Design review of the part shown in the three views and the two pictorial views. Dimensions are in mm from the part's minimum x, y and z. Coordinates: 2 decimals unless noted, no trailing zeros. Loops run counter-clockwise (first coordinate to the right, second up) from the corner with the lowest first, then second, coordinate; pieces in that order, holes last. Notation, with made-up numbers: (-8, -15) -> (-4, -15) arc R19 cw to (-4, 18) -> close; hole circle Ø3 at (30, -26). An arc over 180 degrees is marked (long way). One line per item, written item: value. Start each with the question number.
1. Add section A-A on x = 2.5. Write out the cut boundary in (y, z) (1 decimal), plus the area to 3 significant figures.
2. Insertion check: pin 1 (2 mm diameter, centred on x = 3, z = 16.5, fed in from +Y); pin 2 (8 mm diameter, centred on x = 17.5, z = 10, fed in from +Y); pin 3 (1.5 mm diameter, centred on x = 4.5, z = 15.5, fed in from -Y). Each pin has a flat end and moves straight along its axis. Give the tip position at first contact, or say it passes through.
3. For probe 1 along Z at (x, y) = (19.5, 18); probe 2 along Z at (x, y) = (8.25, 25); probe 3 along Y at (x, z) = (17, 25) (1 decimal), list the stretches that pass through material, from the lowest coordinate up.
4. Draft analysis for pull direction Z (two halves, no side actions). For the marked faces 1, 2, 3 and 4, state which applies: pulls with the +Z half, pulls with the -Z half, needs draft (parallel to the pull), parting line crosses it, or undercut.
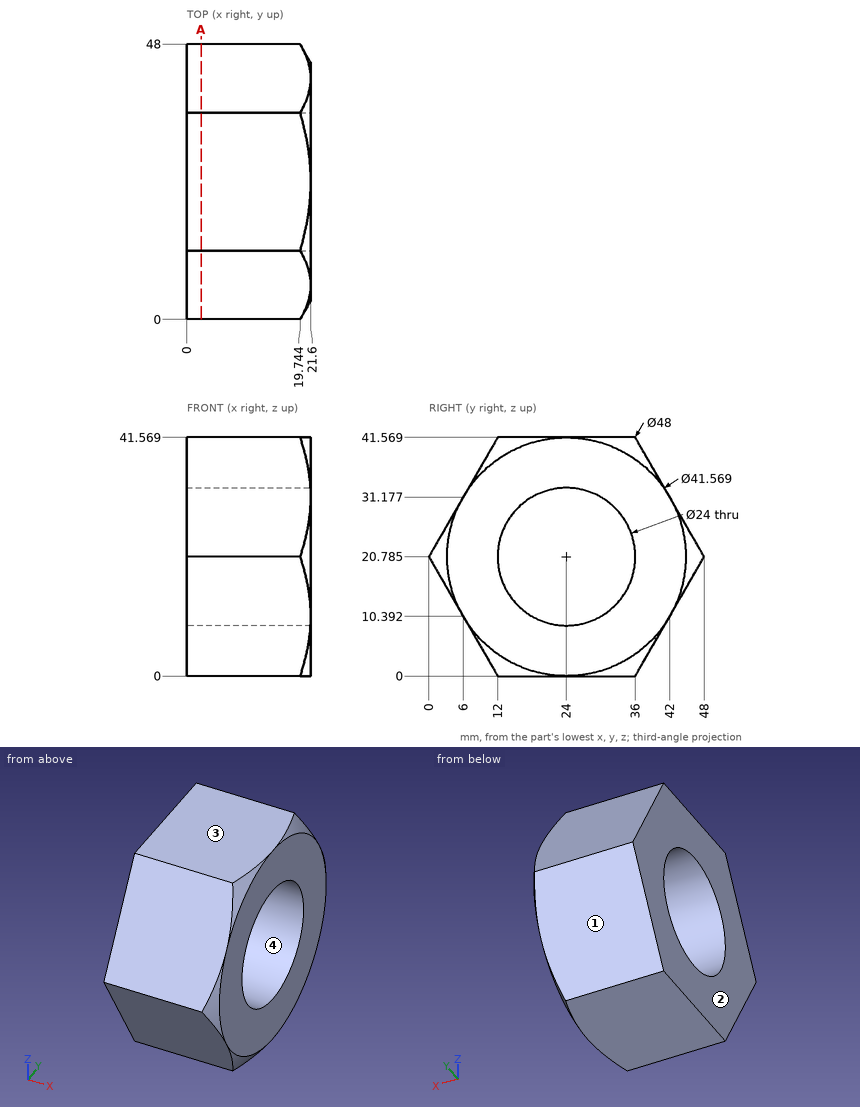
Worked answers:
1. outline: (0, 20.8) -> (12, 0) -> (36, 0) -> (48, 20.8) -> (36, 41.6) -> (12, 41.6) -> close; hole circle Ø24 at (24, 20.8)
1. area: 1,040 mm²
2. pin 1: stops at y = 46.1
2. pin 2: stops at y = 44.08
2. pin 3: stops at y = 2.62
3. probe 1: z = 0 to 10.39, 31.18 to 41.57
3. probe 2: z = 0 to 8.83, 32.74 to 41.57
3. probe 3: y = 2.4 to 12.8, 35.2 to 45.6
4. face 1: pulls with the -Z half
4. face 2: needs draft
4. face 3: pulls with the +Z half
4. face 4: undercut
